Read the model definition and answer for the solid it produces. Units are mm, in the model's axes. Give positions to 0.01 mm unless a question says otherwise; leave off trailing zeros. Order: outer loops, then holes, each group sorted by start corner. A loop starts at its lowest first (then second) coordinate and runs counter-clockwise, first axis right, second up. Notation, with made-up numbers: (-14.75, -24) - (27.25, -24) arc R25 cw to (27.25, 14) - close; hole circle Ø11 at (87.5, 7). An arc over 180 degrees is marked (long way). Return JSON: item names as keys, results as strings.
```python
from build123d import *

# Parameters (mm, degrees)
F0_W      = 129.806437
F0_H      = 123.931572
F1_DEPTH  = 25.4
F1_FACE_W = 129.806436
F1_FACE_H = 123.931572
F2_DEPTH  = 25.4
F3_R      = 6.001171
F4_DEPTH  = 78.486


with BuildPart() as f1:
    # F0 (on Front) → F1 (new body)
    with BuildSketch(Plane.XZ):
        with Locations((-1.258898, 5.035594)):
            Rectangle(F0_W, F0_H)
    extrude(amount=F1_DEPTH)

    # F1_face (on face) → F2 (join)
    with BuildSketch(Plane(origin=(-1.258899, -25.4, 5.035594), x_dir=(1, 0, 0), z_dir=(0, -1, 0))):
        Rectangle(F1_FACE_W, F1_FACE_H)
    extrude(amount=F2_DEPTH)

    # F3 (on face) → F4 (cut)
    with BuildSketch(Plane(origin=(0, 0, 0), x_dir=(-1, 0, 0), z_dir=(0, 1, 0))):
        Circle(F3_R)
    extrude(amount=-F4_DEPTH, mode=Mode.SUBTRACT)


solid = f1.part
```
Q1. A cutting plane is placed at A-A (x = 0). Write down the section's boundary in (y, z), and give its area (3 significant figures).
Values:
{"outline": "(-50.8, -56.93) - (0, -56.93) - (0, -6) - (-50.8, -6) - close; (-50.8, 6) - (0, 6) - (0, 67) - (-50.8, 67) - close", "area": "5,690 mm²"}
Q2. Determine the mould class of faces 1 (the flat face through (63.644, -13, 4)), 2 (the cylindrical face through (-5.724, -25.044, 1.803)), 3 (the flat face through (-2, 0, 6)) for opening direction X: released by +X, released by -X, zero draft, split by the parting line, or undercut.
Values:
{"face 1": "released by +X", "face 2": "undercut", "face 3": "zero draft"}
Q3. Consider L1, parallel to Z at x = 0, y = -17; L2, parallel to Z at x = 2, y = -43.5. Determine where each line is inside the solid, lowest interval first.
Values:
{"L1": "z = -56.93 to -6, 6 to 67", "L2": "z = -56.93 to -5.66, 5.66 to 67"}
